CAD build for the part. Positions are in the model's coordinates, mm. A direction names the side the tool comes from. Give positions to 0.01 mm unless a question says otherwise; leave off trailing zeros. Loops run counter-clockwise (first coordinate to the right, second up) from the corner with the lowest first, then second, coordinate; pieces in that order, holes last. Notation, with made-up numbers: (52.5, 62) - (107.5, 62) arc R24 cw to (107.5, 81) - close; hole circle Ø2 at (-15.75, 50). An arc over 180 degrees is marked (long way). Return JSON: item names as keys, results as strings.
from build123d import *

# Parameters (mm, degrees)
SKETCH1_R                = 4.975
BOSS_EXTRUDE1_DEPTH      = 4
BOSS_EXTRUDE2_START      = 4
SKETCH2_R                = 4.975
BOSS_EXTRUDE2_DEPTH      = 4
BOSS_EXTRUDE5_DEPTH      = 15
BOSS_EXTRUDE5_DEPTH_BACK = 7
SKETCH5_R                = 3.975
CUT_EXTRUDE1_DEPTH       = 17.791552936
CUT_EXTRUDE1_DEPTH_BACK  = 17.791552936
SKETCH9_R                = 1
CHAMFER1_SIZE            = 0.3


with BuildPart() as part:
    # Sketch1 → Boss-Extrude1 (new body)
    with BuildSketch(Plane.XY):
        with Locations((0, 0.7)):
            Circle(SKETCH1_R)
    extrude(amount=BOSS_EXTRUDE1_DEPTH)

    # Sketch2 → Boss-Extrude2 (add)
    with BuildSketch(Plane.XY.offset(BOSS_EXTRUDE2_START)):
        with Locations(Location((0, -0.7, 0), (0, 0, 171.911442188))):
            Circle(SKETCH2_R)
    extrude(amount=BOSS_EXTRUDE2_DEPTH)

    # Sketch5 → Boss-Extrude5 (add, two sides: drawn at the far end of the back side and taken through both)
    with BuildSketch(Plane.XY.offset(-BOSS_EXTRUDE5_DEPTH_BACK)):
        Circle(SKETCH5_R)
    extrude(amount=BOSS_EXTRUDE5_DEPTH + BOSS_EXTRUDE5_DEPTH_BACK)

    # Sketch9 → Cut-Extrude1 (cut, two sides: drawn at the far end of the back side and taken through both)
    with BuildSketch(Plane.XY.offset(-CUT_EXTRUDE1_DEPTH_BACK)):
        with BuildLine():
            ThreePointArc((0, 3.3), (-1, 2.3), (0, 1.3))
            Line((0, 1.3), (0, 3.3))
        make_face()
        with BuildLine():
            Line((0, 3.3), (0, 1.3))
            ThreePointArc((0, 1.3), (0.707106781, 1.592893219), (1, 2.3))
            ThreePointArc((1, 2.3), (0.707106781, 3.007106781), (0, 3.3))
        make_face()
        with Locations((-1.991858429, -1.15)):
            Circle(SKETCH9_R)
        with Locations((1.991858429, -1.15)):
            Circle(SKETCH9_R)
    extrude(amount=CUT_EXTRUDE1_DEPTH + CUT_EXTRUDE1_DEPTH_BACK, mode=Mode.SUBTRACT)

    # Chamfer1
    chamfer1_edges = [part.edges().sort_by_distance(p)[0] for p in [
        (-3.975, 0, 15),
        (0, 1.3, 15),
        (-2.991858429, -1.15, 15),
        (0.991858429, -1.15, 15),
    ]]
    chamfer(chamfer1_edges, length=CHAMFER1_SIZE)


solid = part.part
1. Drop flat-ended pins along their axis: P1, Ø3, axis at x = -1.99, y = -1.15, coming from the +Z side; P2, Ø3, axis at x = -2, z = -2, coming from the +Y side; P3, Ø1, axis at y = -1.5, z = 1.5, coming from the +X side; P4, Ø5, axis at x = 0, z = 11, coming from the +Y side (3 decimals). Give the stop position or say it passes through.
Values follow:
{"P1": "stops at z = 15", "P2": "stops at y = 3.94", "P3": "stops at x = 4.68", "P4": "stops at y = 3.975"}
2. Drill centre lines: probe 1 along X at (y, z) = (-1.15, 1.5); probe 2 along Y at (x, z) = (0, 2.25) (3 decimals); probe 3 along X at (y, z) = (-0.25, 12.25). Where is each one in solid material? Low to high.
Values follow:
{"probe 1": "x = -4.62 to -2.99, -0.99 to 0.99, 2.99 to 4.62", "probe 2": "y = -4.275 to 1.3, 3.3 to 5.675", "probe 3": "x = -3.97 to -2.43, -1.56 to 1.56, 2.43 to 3.97"}
3. Cut at A-A, the plane z = 9. Write the cut outline in (x, y) (3 decimals), plus the area to 3 significant figures.
Values follow:
{"outline": "circle Ø7.95 at (0, 0); hole circle Ø2 at (-1.992, -1.15); hole circle Ø2 at (0, 2.3); hole circle Ø2 at (1.992, -1.15)", "area": "40.2 mm²"}
4. Which spindle directions (+Z, -Z, +X, -X, +Y, -Y) get a long thin tool onto all of the face, cutting with end or side? Do faces 4 (the face through (0, 5, 4)), 5 (the face through (-0.86, -3.88, -3.55)), 6 (the face through (0, -5, 4)), 7 (the face through (0, 0, 15)), 8 (the face through (-2, -4, 8)). Say none if no direction does.
Values follow:
{"face 4": "+Z, +Y", "face 5": "-Z", "face 6": "-Z, -Y", "face 7": "+Z, +X, -X, +Y, -Y", "face 8": "+Z"}
5. Pull direction Y, two halves, no side cores. Call faces 1 (the face through (1.775, -2.126, 3.698)), 2 (the face through (-0.86, -3.88, 11.3)), 3 (the face through (0, 4.4, 0)): +Y half, -Y half, draft (parallel to the pull), parting line (faces both ways), or undercut.
Values follow:
{"face 1": "undercut", "face 2": "parting line", "face 3": "draft"}
6. Cut at D-D, the plane y = -0.7. Give the number of separate pieces and of enclosed holes in the cut face, plus the area to 3 significant figures.
Values follow:
{"separate pieces": "3", "enclosed holes": "0", "area": "109 mm²"}
7. Cut at C-C, the plane y = 4.75. Write the cut outline in (x, z).
Values follow:
{"outline": "(-2.89, 0) - (2.89, 0) - (2.89, 4) - (-2.89, 4) - close"}
8. Cut at B-B, the plane z = 2. Write the cut outline in (x, y) (3 decimals).
Values follow:
{"outline": "circle Ø9.95 at (0, 0.7); hole circle Ø2 at (-1.992, -1.15); hole circle Ø2 at (0, 2.3); hole circle Ø2 at (1.992, -1.15)"}
